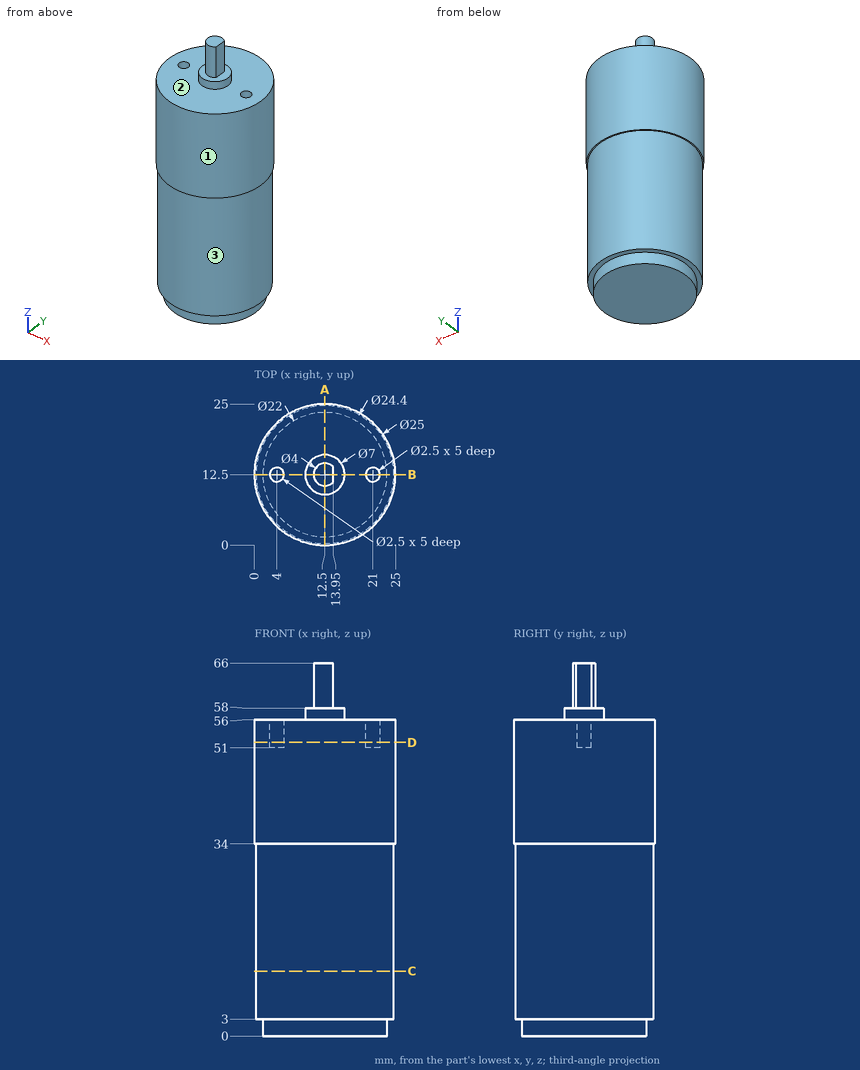
Input: dimensioned drawing with shaded views. Units: mm. Origin: part minimum x, y, z. A direction names the side the tool comes from. Coordinates: 2 decimals unless noted, no trailing zeros. Order: outer loops, then holes, each group sorted by start corner. A loop starts at its lowest first (then second) coordinate and runs counter-clockwise, first axis right, second up.
(1) Section query B-B (y = 12.5). Return the cut outline in (x, z), plus the area to 3 significant figures.
(2) Section query C-C (z = 11.5). Return the cut outline in (x, y), plus the area to 3 significant figures.
(3) Section query D-D (z = 52). Return the cut outline in (x, y).
(4) Access query for the marked faces 1, 2 and 3. Directions: +Z, -Z, +X, -X, +Y, -Y. A direction counts if a zero-diameter tool reaches every point of the face in a straight line with its end or side. Return the directions, or none.
(5) First-contact query: pin 1 (7.5 mm diameter, centred on x = 6.5, y = 18.5, fed in from +Z); pin 2 (1 mm diameter, centred on y = 19.5, z = 37.5, fed in from +X); pin 3 (0.8 mm diameter, centred on x = 4.5, y = 12.5, fed in from +Z). Flat tips, straight axial feed; report the tip coordinate or a pass-through.
(6) Section query A-A (x = 12.5). Return the cut outline in (y, z).
(7) Material intervals for probe 1 along Z at (x, y) = (3, 6.25); probe 2 along Z at (x, y) = (9, 13.75); probe 3 along Y at (x, z) = (4, 53.7), sorted ascending.
Solution:
1. outline: (0, 34) - (0.3, 34) - (0.3, 3) - (1.5, 3) - (1.5, 0) - (23.5, 0) - (23.5, 3) - (24.7, 3) - (24.7, 34) - (25, 34) - (25, 56) - (22.25, 56) - (22.25, 51) - (19.75, 51) - (19.75, 56) - (16, 56) - (16, 58) - (13.95, 58) - (13.95, 66) - (10.5, 66) - (10.5, 58) - (9, 58) - (9, 56) - (5.25, 56) - (5.25, 51) - (2.75, 51) - (2.75, 56) - (0, 56) - close
1. area: 1,390 mm2
2. outline: circle Ø24.4 at (12.5, 12.5)
2. area: 468 mm2
3. outline: circle Ø25 at (12.5, 12.5); hole circle Ø2.5 at (4, 12.5); hole circle Ø2.5 at (21, 12.5)
4. face 1: +Z, -Z
4. face 2: +Z
4. face 3: -Z
5. pin 1: stops at z = 56
5. pin 2: stops at x = 23.18
5. pin 3: stops at z = 51
6. outline: (0, 34) - (0.3, 34) - (0.3, 3) - (1.5, 3) - (1.5, 0) - (23.5, 0) - (23.5, 3) - (24.7, 3) - (24.7, 34) - (25, 34) - (25, 56) - (16, 56) - (16, 58) - (14.5, 58) - (14.5, 66) - (10.5, 66) - (10.5, 58) - (9, 58) - (9, 56) - (0, 56) - close
7. probe 1: z = 3 to 56
7. probe 2: z = 0 to 56
7. probe 3: y = 3.33 to 11.25, 13.75 to 21.67
